Can you work these out from the model? Positions are in its coordinate system, mm. Face numbers are marked on the shaded views. A direction names the side the tool comes from. Coordinates: 2 decimals unless noted, no trailing zeros. Write each loop counter-clockwise with the first axis right and the second up, starting at its lowest first coordinate (ties: lowest second). Pieces come first, ordered by that corner, then holes. Notation, with made-up numbers: (64, -25) -> (90, -25) arc R6 ccw to (90, -20) -> close; hole circle Ø6 at (18.5, 2). An arc over 180 degrees is marked (long way). Use one line per item in the form item = value.
Autodesk Inventor part; units mm, degrees
ref_plane "YZ Plane" through (0, 0, 0) normal (1, 0, 0) x (0, 1, 0)
ref_plane "XZ Plane" through (0, 0, 0) normal (0, 1, 0) x (-1, 0, 0)
ref_plane "XY Plane" through (0, 0, 0) normal (0, 0, 1) x (1, 0, 0)
sketch "Sketch1" plane through (0, 0, 0) normal (0, 0, 1) x (1, 0, 0)
  line L0 (-750, 77.5093) -> (750, 77.5093)
  line L1 (750, 77.5093) -> (750, 0)
  line L2 (750, 0) -> (-750, 0)
  line L3 (-750, 0) -> (-750, 77.5093)
  point P0 (0, 0)
  point P1 (0, 0)
  dimension "d0" = 1500
  dimension "d1" = 77.5093
extrude "Plate1" add sketch "Sketch1" along normal blind 2
sketch "Sketch2" plane through (750, 2, 0) normal (0, -1, 0) x (1, 0, 0)
  line L0 (-1500, 0) -> (0, 0)
  line L1 (0, 0) -> (0, 30)
  line L2 (0, 30) -> (-1500, 30)
  line L3 (-1500, 30) -> (-1500, 0)
edge flange "Flange1" height 30 angle 90 thickness 2 bend radius 2.75 thickness toward (0, -1, 0) relief round relief width 2 relief depth 1 edges at (0, 0, 2) wall of the first edge with corners at (-750, 2, 0) (750, 2, 0) (750, 2, 30) (-750, 2, 30)
bend "Bend1"
corner "Corner1"
sketch "Sketch5" plane through (0, 0, 0) normal (0, 0, -1) x (-1, 0, 0)
  line L0 (750, 77.5093) -> (-750, 77.5093)
  line L1 (-1, 30) -> (-1, 77.5093)
  line L2 (750, 0) -> (-750, 0)
  line L3 (-1, 30) -> (1, 30)
  line L4 (1, 30) -> (1, 77.5093)
  point P0 (0, 0)
  point P1 (0, 30)
  point P2 (0, 0)
  dimension "d27" = 2
  dimension "d28" = 30
extrude "Extrusion1" cut sketch "Sketch5" against normal through all
pattern_linear "Rectangular Pattern1" count 3 spacing 500 along (1, 0, 0) of "Extrusion1" first direction both ways yes
sketch "Sketch6" plane through (0, 0, 0) normal (0, 0, -1) x (-1, 0, 0)
  line L0 (-750, 77.5093) -> (-750, 4.75)
  circle A0 centre (-750, 77.5093) radius 22.5
  line L1 (-750, 77.5093) -> (750, 77.5093)
  line L2 (-1, 77.5093) -> (-1, 30)
  line L3 (-499, 77.5093) -> (-499, 30)
  line L4 (-1, 30) -> (-499, 30) construction
  circle A1 centre (-250, 77.5093) radius 22.5
  point P0 (0, 0)
  point P1 (-727.5, 77.5093)
  point P2 (-750, 55.0093)
  point P3 (-250, 30)
  dimension "d24" = 45
extrude "Extrusion2" cut sketch "Sketch6" along normal mid plane 30 contours L1 A0 L0 | A1 L1 | L1 A1 picked at (-748.3311, 62.6973)
mirror "Mirror1" about plane through (0, 0, 0) normal (1, 0, 0) of "Extrusion2"
sketch "Sketch7" plane through (0, 0, 2) normal (0, 0, 1) x (1, 0, 0)
  arc A0 (-750, 55.0093) -> (-727.5, 77.5093) centre (-750, 77.5093) ccw
  line L0 (-750, 4.75) -> (-750, 55.0093)
  line L1 (-750, 4.75) -> (750, 4.75)
  line L2 (750, 55.0093) -> (750, 4.75)
  arc A1 (727.5, 77.5093) -> (750, 55.0093) centre (750, 77.5093) ccw
  line L3 (501, 77.5093) -> (727.5, 77.5093)
  line L4 (501, 77.5093) -> (501, 30)
  line L5 (501, 30) -> (499, 30)
  line L6 (499, 30) -> (499, 77.5093)
  line L7 (1, 77.5093) -> (227.5, 77.5093)
  line L8 (1, 77.5093) -> (1, 30)
  line L9 (1, 30) -> (-1, 30)
  line L10 (-1, 30) -> (-1, 77.5093)
  line L11 (-499, 77.5093) -> (-272.5, 77.5093)
  line L12 (-499, 77.5093) -> (-499, 30)
  line L13 (-499, 30) -> (-501, 30)
  line L14 (-501, 30) -> (-501, 77.5093)
  line L15 (-727.5, 77.5093) -> (-501, 77.5093)
  line L16 (750, 4.75) -> (-750, 4.75)
  line L17 (650, 4.75) -> (650, 77.5093) construction
  line L18 (-750, 4.75) -> (750, 4.75)
  line L19 (646, 37.6655) -> (650, 44.5938)
  line L20 (650, 44.5938) -> (654, 37.6655)
  line L21 (654, 37.6655) -> (646, 37.6655)
  line L22 (650, 44.5938) -> (650, 37.6655) construction
  line L23 (626, 37.6655) -> (630, 44.5938)
  line L24 (630, 44.5938) -> (634, 37.6655)
  line L25 (634, 37.6655) -> (626, 37.6655)
  line L26 (630, 44.5938) -> (630, 37.6655) construction
  line L27 (272.5, 77.5093) -> (499, 77.5093)
  arc A2 (227.5, 77.5093) -> (272.5, 77.5093) centre (250, 77.5093) ccw
  line L28 (-227.5, 77.5093) -> (-1, 77.5093)
  arc A3 (-272.5, 77.5093) -> (-227.5, 77.5093) centre (-250, 77.5093) ccw
  point P0 (0, 0)
  point P1 (650, 41.1296)
  point P2 (630, 41.1296)
  dimension "d29" = 100
  dimension "d30" = 8
  dimension "d31" = 8
  dimension "d32" = 20
extrude "Extrusion3" [suppressed]
mirror "Mirror2" [suppressed]
sketch "Sketch8" plane through (0, 0, 2) normal (0, 0, 1) x (1, 0, 0)
  line L0 (496, 72.5093) -> (496, 60.5093) construction
  line L1 (496, 60.5093) -> (296, 60.5093) construction
  line L2 (296, 60.5093) -> (296, 72.5093) construction
  line L3 (296, 72.5093) -> (496, 72.5093) construction
  line L4 (501, 77.5093) -> (727.5, 77.5093)
  line L5 (272.5, 77.5093) -> (499, 77.5093)
  point P0 (0, 0)
  dimension "d35" = 200
  dimension "d36" = 12
  dimension "d39" = 3
  dimension "d40" = 5
mark "Mark1"
equation "\"d1\" = Стрингер_6"
equation "\"d27\" = d18"
equation "\"d2\" = Thickness"
equation "\"d3\" = BendReliefWidth"
equation "\"d4\" = BendReliefDepth"
equation "\"d5\" = MinimumRemnant"
equation "\"d6\" = TransitionRadius"
equation "\"d9\" = BendRadius"
equation "\"d10\" = CornerReliefSize"
equation "\"d11\" = GapSize"
equation "\"d12\" = JacobiRadiusSize"
equation "\"BendReliefWidth\" = Thickness"
equation "\"BendReliefDepth\" = 0.5 * Thickness"
equation "\"CornerReliefSize\" = 4 * Thickness"
equation "\"MinimumRemnant\" = 2 * Thickness"
equation "\"TransitionRadius\" = BendRadius"
equation "\"JacobiRadiusSize\" = BendRadius"
equation "\"GapSize\" = Thickness"
equation "\"d18\" = Thickness"
properties part number "MSC 066 stringer board ####" material "Stainless Steel"
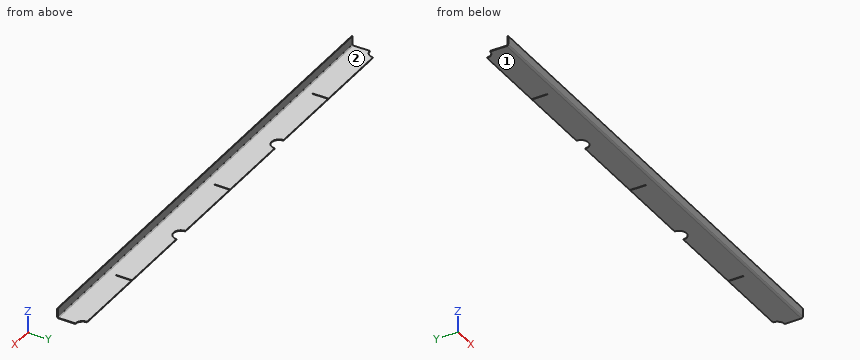
Q1. Suppose I cut it at B-B (y = 17.5). Write out the boundary of the cut face in (x, z), then the cut area to 3 significant figures.
Return value:
outline = (-750, 0) -> (750, 0) -> (750, 2) -> (-750, 2) -> close
area = 3,000 mm2
Q2. Suppose I cut it at A-A (x = -649). Write out the boundary of the cut face in (y, z).
Return value:
outline = (0, 4.75) arc R4.75 ccw to (4.75, 0) -> (77.51, 0) -> (77.51, 2) -> (4.75, 2) arc R2.75 cw to (2, 4.75) -> (2, 30) -> (0, 30) -> close
Q3. Suppose I cut it at C-C (x = -250). Write out the boundary of the cut face in (y, z).
Return value:
outline = (0, 4.75) arc R4.75 ccw to (4.75, 0) -> (55.01, 0) -> (55.01, 2) -> (4.75, 2) arc R2.75 cw to (2, 4.75) -> (2, 30) -> (0, 30) -> close
Q4. If I drill on line 1 (Z direction, x = -287, y = 14.5); line 2 (Y direction, x = -71, z = 3), over which ranges is the centre line in solid material (lowest first)? Write a range as from..to.
Return value:
line_1 = 0..2
line_2 = 0.33..2.63
Q5. Will these pins go through, and if not, where does the flat tip stop? pin 1 (2 mm diameter, centred on x = 80, y = 52.5, fed in from -Z); pin 2 (0.6 mm diameter, centred on y = 65.5, z = 1, fed in from -X); pin 3 (3 mm diameter, centred on x = -463.5, y = 66.5, fed in from +Z); pin 4 (1 mm diameter, centred on y = 64, z = 0.5, fed in from -X).
Return value:
pin_1 = 0
pin_2 = -731.17
pin_3 = 2
pin_4 = -732.39
Q6. For the marked faces 1 and 2, which set-ups out of +Z, -Z, +X, -X, +Y, -Y let a thin tool reach every point of the face, with its end or its side?
Return value:
face_1 = -Z, +X, -X, +Y, -Y
face_2 = +Z, +X, -X, +Y
